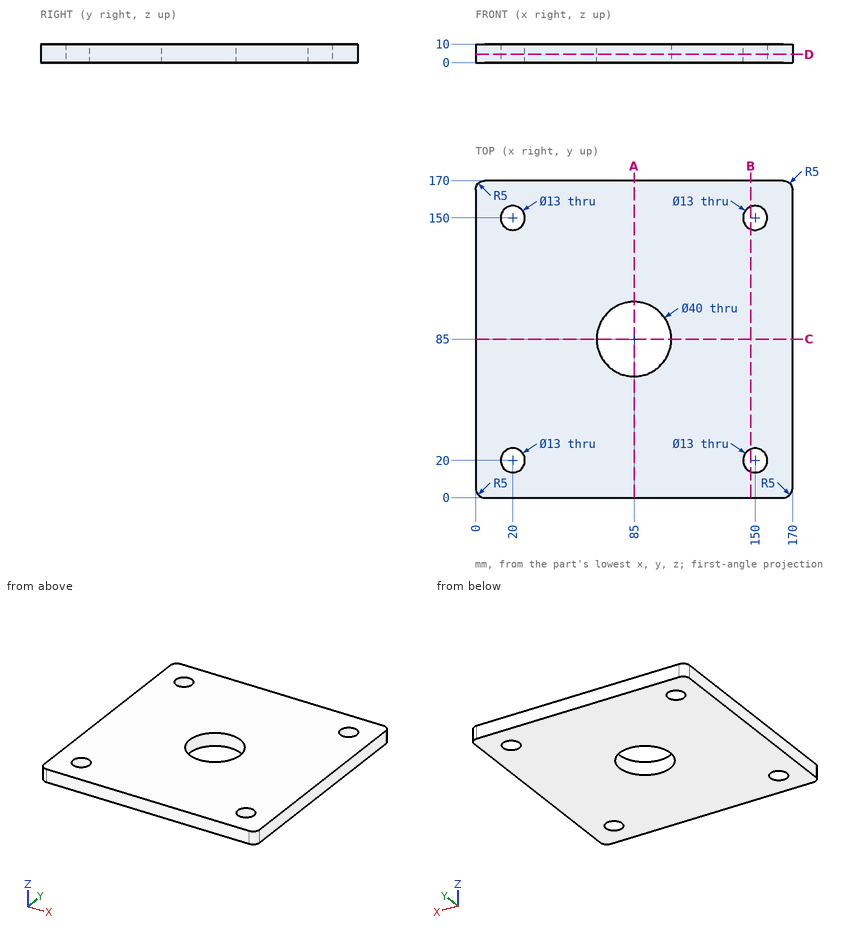
Print and shaded views of the part. All mm, measured from the part's lowest x, y and z. Coordinates: 2 decimals unless noted, no trailing zeros. Write each loop counter-clockwise with the first axis right and the second up, starting at its lowest first coordinate (ties: lowest second). Pieces come first, ordered by that corner, then holes. Notation, with made-up numbers: M -26.75,25.25 L -2.75,25.25 A6 ccw -2.75,30.25 Z; hole C 4.5,-17.75 d1. An arc over 180 degrees is marked long. Return JSON: item names as keys, results as strings.
1. Flat gauge pin, fed straight in: pin 1 Ø8 at (x, y) = (20, 20) entering from -Z. Where does the tip first touch, or does it go through?
Determined:
{"pin 1": "through"}
2. Saw through at D-D, the plane z = 4.5. Write the cut outline in (x, y), then the cut area to 3 significant figures.
Determined:
{"outline": "M 0,5 A5 ccw 5,0 L 165,0 A5 ccw 170,5 L 170,165 A5 ccw 165,170 L 5,170 A5 ccw 0,165 Z; hole C 20,20 d13; hole C 20,150 d13; hole C 85,85 d40; hole C 150,20 d13; hole C 150,150 d13", "area": "27,100 mm²"}
3. Saw through at A-A, the plane x = 85. Write the cut outline in (y, z).
Determined:
{"outline": "M 0,0 L 65,0 L 65,10 L 0,10 Z; M 105,0 L 170,0 L 170,10 L 105,10 Z"}
4. Saw through at B-B, the plane x = 147.5. Write the cut outline in (y, z).
Determined:
{"outline": "M 0,0 L 14,0 L 14,10 L 0,10 Z; M 26,0 L 144,0 L 144,10 L 26,10 Z; M 156,0 L 170,0 L 170,10 L 156,10 Z"}
5. Probe L1, parallel to Y at x = 20, z = 2; L2, parallel to X at y = 144, z = 2.5; L3, parallel to X at y = 18, z = 6. List the from-to ranges inside material, lowest first.
Determined:
{"L1": "0 to 13.5, 26.5 to 143.5, 156.5 to 170", "L2": "0 to 17.5, 22.5 to 147.5, 152.5 to 170", "L3": "0 to 13.82, 26.18 to 143.82, 156.18 to 170"}
